from build123d import *

# Parameters (mm, degrees)
F0_W     = 18.1465977803
F0_H     = 77.7187608182
F1_DEPTH = 7.62
F3_DEPTH = 25.4
F4_R     = 3.7710052393
F4_R_2   = 4.2515891663
F5_DEPTH = 25.4


with BuildPart() as f1:
    # F0 (on Top) → F1 (new body)
    with BuildSketch(Plane.XY):
        with Locations((-18.3298974298, -4.2158756405)):
            Rectangle(F0_W, F0_H)
    extrude(amount=F1_DEPTH)

    # F2 (on face) → F3 (cut)
    with BuildSketch(Plane.XY.offset(7.62)):
        with BuildLine():
            ThreePointArc((-27.4031963199, 25.4119987424), (-18.5065865257, 34.3413978482), (-9.2565985397, 25.7785971101))
            Line((-9.2565985397, 25.7785971101), (-9.2565985397, 34.6435047686))
            Line((-9.2565985397, 34.6435047686), (-27.4031963199, 34.6435047686))
            Line((-27.4031963199, 34.6435047686), (-27.4031963199, 25.4119987424))
        make_face()
        with BuildLine():
            Line((-27.4031963199, -43.0752560496), (-21.1813880653, -43.0752560496))
            ThreePointArc((-21.1813880653, -43.0752560496), (-25.3327232093, -40.2921749844), (-27.4031963199, -35.7432998717))
            Line((-27.4031963199, -35.7432998717), (-27.4031963199, -43.0752560496))
        make_face()
        with BuildLine():
            Line((-9.2565985397, -43.0752560496), (-9.2565985397, -35.376701504))
            ThreePointArc((-9.2565985397, -35.376701504), (-11.2569593187, -40.150009887), (-15.526485177, -43.0752560496))
            Line((-15.526485177, -43.0752560496), (-9.2565985397, -43.0752560496))
        make_face()
    extrude(amount=-F3_DEPTH, mode=Mode.SUBTRACT)

    # F4 (on face) → F5 (cut)
    with BuildSketch(Plane.XY.offset(7.62)):
        with Locations((-18.3539366212, -34.3700621202)):
            Circle(F4_R)
        with Locations((-18.4215474874, 21.0793800652)):
            Circle(F4_R_2)
    extrude(amount=-F5_DEPTH, mode=Mode.SUBTRACT)


solid = f1.part
Could you check a few things on this model? Use its own coordinates, in mm. Give positions to 0.01 mm unless a question says otherwise; leave off trailing zeros. Write each loop counter-clockwise with the first axis right and the second up, starting at its lowest first coordinate (ties: lowest second). Pieces come first, ordered by that corner, then holes. Notation, with made-up numbers: (40.5, 22) -> (71.5, 22) arc R25 cw to (71.5, 60) -> close; hole circle Ø10 at (66.5, 73). An arc over 180 degrees is marked (long way). Write each question's results on one line, items separated by ' | '. Start each with the question number.
Q1. Suppose I cut it at A-A, the plane y = 23. List the corners of the cut face in (x, z) for me.
Q2. Suppose I cut it at C-C, the plane z = 6.5. List the corners of the cut face in (x, y) for me, and give its area (3 significant figures).
Q3. I need wall thicknesses on probe 1 along X at (y, z) = (21, 6.25); probe 2 along Y at (x, z) = (-18, 3.75); probe 3 along Y at (x, z) = (-16, 7.25). Which ranges of each line are inside material? Lowest first, please.
Q4. I'm going to push flat-ended pins straight in: pin 1 Ø1.5 at (x, z) = (-13, 6) entering from -Y; pin 2 Ø4 at (x, z) = (-11.5, 2) entering from +Y; pin 3 Ø5 at (x, y) = (-18.42, 21.08) entering from +Z; pin 4 Ø1.5 at (x, z) = (-22, 3.5) entering from -Y. Where does each tip first touch, or does it pass through?
Q5. Suppose I cut it at D-D, the plane x = -25. List the corners of the cut face in (y, z) for me.
Q6. Suppose I cut it at B-B, the plane x = -16.5. List the corners of the cut face in (y, z) for me.
Q7. We'd pull the mould along X, two halves only. Please class faces 1 (the face through (-25.287, -40.346, 3.863)), 2 (the face through (-14.87, -35.81, 3.86)), 3 (the face through (-18, -43.075, 4)): +X half, -X half, draft (parallel to the pull), parting line (faces both ways), or undercut.
Outcome:
1) outline: (-27.4, 0) -> (-22.21, 0) -> (-22.21, 7.62) -> (-27.4, 7.62) -> close; (-14.63, 0) -> (-9.26, 0) -> (-9.26, 7.62) -> (-14.63, 7.62) -> close
2) outline: (-27.4, -35.74) arc R9.15 ccw to (-21.18, -43.08) -> (-15.53, -43.08) arc R9.15 ccw to (-9.26, -35.38) -> (-9.26, 25.78) arc R9.08 ccw to (-27.4, 25.41) -> close; hole circle Ø8.5 at (-18.42, 21.08); hole circle Ø7.54 at (-18.35, -34.37) | area: 1,240 mm2
3) probe 1: -27.4 to -22.67, -14.17 to -9.26 | probe 2: -43.08 to -38.12, -30.62 to 16.85, 25.31 to 34.34 | probe 3: -43.08 to -37.32, -31.42 to 17.58, 24.57 to 34.04
4) pin 1: y = -42.28 | pin 2: y = 32.96 | pin 3: through | pin 4: y = -43.05
5) outline: (-40.66, 0) -> (31.42, 0) -> (31.42, 7.62) -> (-40.66, 7.62) -> close
6) outline: (-43.08, 0) -> (-37.65, 0) -> (-37.65, 7.62) -> (-43.08, 7.62) -> close; (-31.09, 0) -> (17.29, 0) -> (17.29, 7.62) -> (-31.09, 7.62) -> close; (24.87, 0) -> (34.16, 0) -> (34.16, 7.62) -> (24.87, 7.62) -> close
7) face 1: -X half | face 2: undercut | face 3: draft
